Can you work these out from the drawing? Everything is in mm from the part's minimum corner. A direction names the side the tool comes from. Give positions to 0.01 mm unless a question says otherwise; leave off trailing zeros. Write each loop counter-clockwise with the first axis right and the second up, starting at its lowest first coordinate (ties: lowest second). Pieces come first, ordered by that corner, then holes. Notation, with made-up numbers: (12, 35) -> (59, 35) arc R16 cw to (59, 46) -> close; hole circle Ø2 at (-27.5, 59). An arc over 180 degrees is marked (long way). Use one line per item in the form item = value.
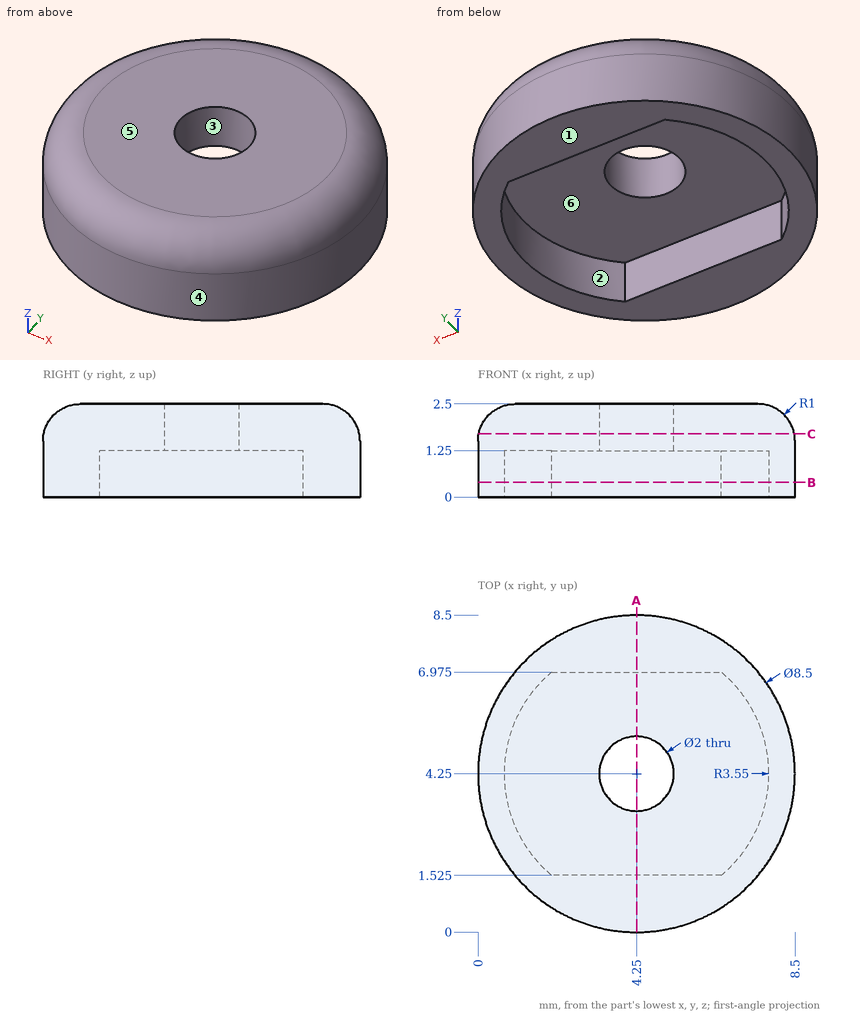
Q1. Will these pins go through, and if not, where does the flat tip stop? pin 1 Ø2 at (x, y) = (4.5, 2) entering from -Z; pin 2 Ø1 at (x, z) = (5, 0.5) entering from -Y.
Result set:
pin_1 = 0
pin_2 = 0.01
Q2. I want a section at B-B, the plane z = 0.4. Write out the boundary of the cut face in (x, y) (3 decimals).
Result set:
outline = circle Ø8.5 at (4.25, 4.25); hole (1.975, 1.525) -> (6.525, 1.525) arc R3.55 ccw to (6.525, 6.975) -> (1.975, 6.975) arc R3.55 ccw to start
Q3. Which directions (+Z, -Z, +X, -X, +Y, -Y) give clear straight access to the entire face, cutting with the end or side of a thin tool? Please do the marked faces 5 and 6.
Result set:
face_5 = +Z, +X, -X, +Y, -Y
face_6 = -Z
Q4. I want a section at C-C, the plane z = 1.7. Write out the boundary of the cut face in (x, y), and give its area (3 significant figures).
Result set:
outline = circle Ø8.46 at (4.25, 4.25); hole circle Ø2 at (4.25, 4.25)
area = 53.1 mm2
Q5. I want a section at A-A, the plane x = 4.25. Write out the boundary of the cut face in (y, z) (3 decimals), and give its area (3 significant figures).
Result set:
outline = (0, 0) -> (1.525, 0) -> (1.525, 1.25) -> (3.25, 1.25) -> (3.25, 2.5) -> (1, 2.5) arc R1 ccw to (0, 1.5) -> close; (5.25, 1.25) -> (6.975, 1.25) -> (6.975, 0) -> (8.5, 0) -> (8.5, 1.5) arc R1 ccw to (7.5, 2.5) -> (5.25, 2.5) -> close
area = 11.5 mm2
Q6. If we mould it in two halves opening along X, with no side actions, what happens to the marked faces 1, 2, 3 and 4? For each: +X half, -X half, draft (parallel to the pull), parting line (faces both ways), or undercut.
Result set:
face_1 = draft
face_2 = undercut
face_3 = undercut
face_4 = parting line
Q7. If I drill on line 1 along Y through (x, z) = (2.75, 0.85) (1 decimal); line 2 along Z through (x, y) = (3, 6); line 3 along Y through (x, z) = (4.5, 1.95), over which ranges is the centre line in solid material (lowest first)? Write a range as from..to.
Result set:
line_1 = 0.3..1.5, 7..8.2
line_2 = 1.25..2.5
line_3 = 0.11..3.28, 5.22..8.39
